from build123d import *

# Parameters (mm, degrees)
SKETCH1_R           = 15.5
BOSS_EXTRUDE1_DEPTH = 0.5
BOSS_EXTRUDE2_DEPTH = 1
FILLET1_R           = 1.25


with BuildPart() as part:
    # Sketch1 → Boss-Extrude1 (new body)
    with BuildSketch(Plane.XY):
        Circle(SKETCH1_R)
    extrude(amount=BOSS_EXTRUDE1_DEPTH)

    # Sketch2 → Boss-Extrude2 (add)
    with BuildSketch(Plane.XY.offset(0.5)):
        Polygon((-11.907849302, -6.875), (11.907849302, -6.875), (0, 13.75), align=None)
    extrude(amount=BOSS_EXTRUDE2_DEPTH)

    # Fillet1
    fillet1_edges = [part.edges().sort_by_distance(p)[0] for p in [
        (0, 13.75, 1),
        (-11.907849302, -6.875, 1),
        (11.907849302, -6.875, 1),
    ]]
    fillet(fillet1_edges, radius=FILLET1_R)


solid = part.part
Read the model definition and answer for the solid it produces. Units are mm, in the model's axes. A direction names the side the tool comes from. Round coordinates to 2 decimals unless told otherwise and drop trailing zeros. Write each loop counter-clockwise with the first axis right and the second up, starting at its lowest first coordinate (ties: lowest second). Pieces come first, ordered by that corner, then holes.
1. The part is cut by section C-C, the plane z = 1.2. Determine the outline of the cut face in (x, y) (3 decimals).
2. Which of the six approach directions +Z, -Z, +X, -X, +Y, -Y give full straight-line access (tool end or side, diameter ignored) to faces 1 (the face through (0, 12.5, 1)), 2 (the face through (7, 4, 0.5)), 3 (the face through (0, -6.875, 1)), 4 (the face through (-10.816, -6.266, 1.007))?
3. Given pin 1 Ø2 at (x, y) = (7, -11) entering from -Z; pin 2 Ø0.5 at (x, z) = (3.5, 1) entering from -Y (3 decimals); pin 3 Ø2 at (x, y) = (-8.5, 9.5) entering from +Z, each flat-ended and moving along its own axis, determine where each tip first touches the part or whether it passes through.
4. The part is cut by section B-B, the plane y = 1.5. Determine the outline of the cut face in (x, z).
5. The part is cut by section A-A, the plane x = 0. Determine the outline of the cut face in (y, z) (3 decimals), then the cut area to 3 significant figures.
6. Straight lines are drawn through the part: L1, parallel to Z at x = 4, y = -7; L2, parallel to X at y = -0.5, z = 0.95; L3, parallel to Y at x = 1, z = 1.45 (3 decimals). For each, find the intervals that lie inside material, in ascending order.
Values:
1. outline: (-10.825, -5) arc R1.25 ccw to (-9.743, -6.875) - (9.743, -6.875) arc R1.25 ccw to (10.825, -5) - (1.083, 11.875) arc R1.25 ccw to (-1.083, 11.875) - close
2. face 1: +Z, +Y
2. face 2: +Z
2. face 3: +Z, +X, -X, -Y
2. face 4: +Z, -X
3. pin 1: stops at z = 0
3. pin 2: stops at y = -6.875
3. pin 3: stops at z = 0.5
4. outline: (-15.43, 0) - (15.43, 0) - (15.43, 0.5) - (7.07, 0.5) - (7.07, 1.5) - (-7.07, 1.5) - (-7.07, 0.5) - (-15.43, 0.5) - close
5. outline: (-15.5, 0) - (15.5, 0) - (15.5, 0.5) - (12.5, 0.5) - (12.5, 1.5) - (-6.875, 1.5) - (-6.875, 0.5) - (-15.5, 0.5) - close
5. area: 34.9 mm2
6. L1: z = 0 to 0.5
6. L2: x = -8.23 to 8.23
6. L3: y = -6.875 to 12
